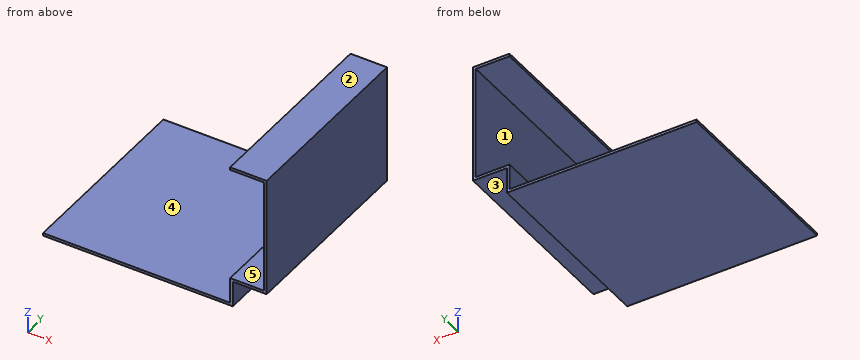
from build123d import *

# Parameters (mm, degrees)
F1_DEPTH = 33.5
F2_W     = 83
F2_H     = 1.2
F3_DEPTH = 42.5
F5_DEPTH = 76.001
F7_DEPTH = 76.001


with BuildPart() as f1:
    # F0 (on Front) → F1 (new body, symmetric)
    with BuildSketch(Plane.XZ):
        Polygon((83, 0), (0, 0), (0, -23), (83, -23), (83, -11.5), align=None)
        Polygon((83, 39), (83, 0), (83, -11.5), (98, -11.5), (98, 39), align=None)
    extrude(amount=F1_DEPTH, both=True)

    # F2 (on Front) → F3 (join, symmetric)
    with BuildSketch(Plane.XZ):
        Polygon((83, 40.2), (83, 39), (98, 39), (99.2, 39), (99.2, 40.2), align=None)
        Polygon((99.2, 39), (98, 39), (98, -11.5), (98, -12.7), (99.2, -12.7), align=None)
        with Locations((41.5, -23.6)):
            Rectangle(F2_W, F2_H)
        Polygon((83, -12.7), (83, -23), (83, -24.2), (84.2, -24.2), (84.2, -12.7), align=None)
        Polygon((98, -12.7), (98, -11.5), (83, -11.5), (83, -12.7), (84.2, -12.7), align=None)
    extrude(amount=F3_DEPTH, both=True)

    # F4 (on face) → F5 (cut, through all)
    with BuildSketch(Plane.XZ.offset(33.5)):
        Polygon((21, -21), (2, -2), (2, -21), align=None)
        Polygon((21.848528, -20.151472), (40, -2), (3.697056, -2), align=None)
        Polygon((40.848528, -2.848528), (22.697056, -21), (59, -21), align=None)
        Polygon((59.848528, -20.151472), (78, -2), (41.697056, -2), align=None)
        Polygon((81, -9.5), (85.5, -9.5), (78.848528, -2.848528), (60.697056, -21), (81, -21), align=None)
        Polygon((96, -9.5), (96, 0), (86.286385, -8.788509), (86.997877, -9.5), align=None)
        Polygon((96, 2.302944), (85, 13.302944), (85, -2), (79.497877, -2), (85.436797, -7.93892), (96, 1.618263), align=None)
        Polygon((96, 4), (96, 24.302944), (85.848528, 14.151472), align=None)
        Polygon((95.151472, 25.151472), (85, 35.302944), (85, 15), align=None)
        Polygon((96, 37), (85, 37), (96, 26), align=None)
    extrude(amount=-F5_DEPTH, mode=Mode.SUBTRACT)

    # F6 (on face) → F7 (cut, through all)
    with BuildSketch(Plane.XZ.offset(33.5)):
        Polygon((83, 39), (83, 0), (0, 0), (0, -23), (83, -23), (83, -11.5), (98, -11.5), (98, 39), align=None)
    extrude(amount=-F7_DEPTH, mode=Mode.SUBTRACT)


solid = f1.part
Source: CAD feature listing. Evaluate the final solid. Frame: model axes, mm. Face numbers are marked on the shaded views. A direction names the side the tool comes from. Give positions to 0.01 mm unless a question says otherwise; leave off trailing zeros. Write each loop counter-clockwise with the first axis right and the second up, starting at its lowest first coordinate (ties: lowest second). Pieces come first, ordered by that corner, then holes. Notation, with made-up numbers: (-2.75, 69.25) - (46.25, 69.25) arc R27 ccw to (46.25, 104.25) - close; hole circle Ø1 at (-1.5, -28). An arc over 180 degrees is marked (long way). Write item = value, one per line. Start each with the question number.
Q1. Pin query (flat end, axial travel): pin 1 Ø16.5 at (x, y) = (94.5, -8) entering from -Z; pin 2 Ø5 at (y, z) = (1.5, -14) entering from -X; pin 3 Ø4 at (x, y) = (41.5, -8.5) entering from +Z. Return the tip coordinate at first contact, or that it passes through.
Q2. Cut plane C-C, the plane z = -15. Return loops of the section in (x, y), then the cut area to 3 significant figures.
Q3. Reachability of the marked faces 1 and 2 from +Z, -Z, +X, -X, +Y, -Y: full face, straight path, thin tool, end or side. Return the list, or none.
Q4. Cut plane B-B, the plane x = 33. Return loops of the section in (y, z), then the cut area to 3 significant figures.
Q5. Material intervals for probe 1 along Z at (x, y) = (94, 28); probe 2 along X at (y, z) = (17, 4); probe 3 along X at (y, z) = (19.5, -17), sorted ascending.
Q6. Draft query along Z for the marked faces 3, 4 and 5. Return one class per face: +Z half, -Z half, draft (parallel to the pull), parting line (faces both ways), or undercut.
Q7. Cut plane A-A, the plane y = 7. Return loops of the section in (x, z), then the cut area to 3 significant figures.
Computed values:
q1.pin_1 = -12.7
q1.pin_2 = 83
q1.pin_3 = -23
q2.outline = (83, -42.5) - (84.2, -42.5) - (84.2, 42.5) - (83, 42.5) - close
q2.area = 102 mm²
q3.face_1 = -X, +Y, -Y
q3.face_2 = +Z, +X, -X, +Y, -Y
q4.outline = (-42.5, -24.2) - (42.5, -24.2) - (42.5, -23) - (-42.5, -23) - close
q4.area = 102 mm²
q5.probe_1 = -12.7 to -11.5, 39 to 40.2
q5.probe_2 = 98 to 99.2
q5.probe_3 = 83 to 84.2
q6.face_3 = -Z half
q6.face_4 = +Z half
q6.face_5 = undercut
q7.outline = (0, -24.2) - (84.2, -24.2) - (84.2, -12.7) - (99.2, -12.7) - (99.2, 40.2) - (83, 40.2) - (83, 39) - (98, 39) - (98, -11.5) - (83, -11.5) - (83, -23) - (0, -23) - close
q7.area = 213 mm²
